Work out the finished part from the listing and answer in its coordinate system (mm). A direction names the side the tool comes from. Round coordinates to 2 decimals unless told otherwise and drop trailing zeros. Write each loop counter-clockwise with the first axis right and the second up, starting at its lowest first coordinate (ties: lowest second). Pieces come first, ordered by that corner, then holes. Notation, with made-up numbers: (20.25, 71.5) - (67.25, 71.5) arc R25 ccw to (67.25, 95.5) - close; hole circle Ø9 at (43, 33.25). An arc over 180 degrees is marked (long way). Answer as a JSON object with one key per item and string values.
Autodesk Inventor part; units mm, degrees
ref_plane "YZ Plane" through (0, 0, 0) normal (1, 0, 0) x (0, 1, 0)
ref_plane "XZ Plane" through (0, 0, 0) normal (0, 1, 0) x (-1, 0, 0)
ref_plane "XY Plane" through (0, 0, 0) normal (0, 0, 1) x (1, 0, 0)
sketch "Sketch1" plane through (0, 0, 0) normal (1, 0, 0) x (0, 1, 0)
  line L0 (-7.4638, 10.773) -> (-7.4638, 13.3671)
  line L1 (-0.652, 13.3671) -> (-0.652, 10.773)
  arc A0 (-0.652, 13.3671) -> (-7.4638, 13.3671) centre (-4.0579, 13.3671) ccw
  line L2 (0.948, 10.773) -> (0.948, 13.3671)
  arc A1 (0.948, 13.3671) -> (-9.0638, 13.3671) centre (-4.0579, 13.3671) ccw
  line L3 (-9.0638, 13.3671) -> (-9.0638, 10.773)
  line L4 (-9.0638, 10.773) -> (-7.4638, 10.773)
  line L5 (-0.652, 10.773) -> (-0.652, -6.227)
  line L6 (-4.0579, 16.773) -> (-4.0579, 10.773)
  line L7 (0.948, 10.773) -> (0.948, -6.227)
  line L8 (-0.652, 2.273) -> (-9.3077, 2.273)
  line L9 (-7.4638, -6.227) -> (-7.4638, -8.8211)
  line L10 (-0.652, -8.8211) -> (-0.652, -6.227)
  arc A2 (-7.4638, -8.8211) -> (-0.652, -8.8211) centre (-4.0579, -8.8211) ccw
  line L11 (0.948, -6.227) -> (0.948, -8.8211)
  arc A3 (-9.0638, -8.8211) -> (0.948, -8.8211) centre (-4.0579, -8.8211) ccw
  line L12 (-9.0638, -8.8211) -> (-9.0638, -6.227)
  line L13 (0.948, -6.227) -> (0.948, 10.773)
  line L14 (-9.0638, -6.227) -> (-7.4638, -6.227)
  point P0 (0, 0)
  point P1 (0.948, -6.227)
  dimension "d3" = 1.6
  dimension "d4" = 17
  dimension "d5" = 6
extrude "Extrusion1" add sketch "Sketch1" along normal blind 10
sketch "Sketch2" plane through (0, 0.948, 13.3671) normal (0, 1, 0) x (1, 0, 0)
  line L0 (0, 22.1882) -> (0, 0)
  line L1 (0, 0) -> (10, 0)
  line L2 (10, 22.1882) -> (10, 0)
  line L3 (0, 22.1882) -> (10, 22.1882)
  point P0 (0, 13.3671)
  point P1 (5, 11.0941)
  point P2 (0, 11.0941)
  point P3 (5, 0)
hole "Hole1" at (5, 0.948, 2.273) direction (0, -1, 0) diameter 3 end through all countersink diameter 6 countersink angle 90
properties part number "klips"
Item 1: Consider line 1 along Y through (x, z) = (5.5, -6.5); line 2 along Z through (x, y) = (6, -7.75); line 3 along Z through (x, y) = (5, -0.6). Determine where each line is inside the solid, lowest interval first.
Results found:
{"line 1": "-9.06 to -7.46, -0.65 to 0.95", "line 2": "-12.2 to -6.23, 10.77 to 16.75", "line 3": "-12.44 to 0.77, 3.77 to 16.99"}
Item 2: Determine the mould class of faces 1 (the cylindrical face through (4.93, -4.17, 18.37)), 2 (the cylindrical face through (4.93, -3.983, -12.226)), 3 (the flat face through (5, -7.464, 12)), 4 (the flat face through (2.7, 0.948, -0.3)) for opening direction Z: pulls with the +Z half, pulls with the -Z half, needs draft (parallel to the pull), parting line crosses it, or undercut.
Results found:
{"face 1": "pulls with the +Z half", "face 2": "undercut", "face 3": "undercut", "face 4": "needs draft"}
Item 3: Each of these flat-tipped pins is pushed along its axis until it touches: P1, Ø1.3, axis at x = 6, y = -8.5, coming from the +Z side (3 decimals); P2, Ø5, axis at x = 5, z = 2.273, coming from the +Y side; P3, Ø1.3, axis at x = 2.5, y = -8.5, coming from the -Z side. Where does it stop, or does it pass through?
Results found:
{"P1": "z = 16.635", "P2": "y = 0.45", "P3": "z = -12.09"}
Item 4: A cutting plane is placed at B-B (z = -7.5). Write down the section's boundary in (x, y).
Results found:
{"outline": "(0, -9.06) - (10, -9.06) - (10, -7.46) - (0, -7.46) - close; (0, -0.65) - (10, -0.65) - (10, 0.95) - (0, 0.95) - close"}
Item 5: For faces 5 (the cylindrical face through (4.93, -4.133, 16.772)), 6 (the flat face through (5, -9.064, -8)), 7 (the flat face through (5, -8, -6.227)), determine the directions among +Z, -Z, +X, -X, +Y, -Y from which every point of the face is accessible in a straight line to the end or side of a thin tool.
Results found:
{"face 5": "+X, -X", "face 6": "+Z, -Z, +X, -X, -Y", "face 7": "+X, -X, -Y"}
Item 6: A cutting plane is placed at D-D (y = -1.5). Write down the section's boundary in (x, z).
Results found:
{"outline": "(0, -13.12) - (10, -13.12) - (10, -11.07) - (0, -11.07) - close; (0, 15.62) - (10, 15.62) - (10, 17.67) - (0, 17.67) - close"}
